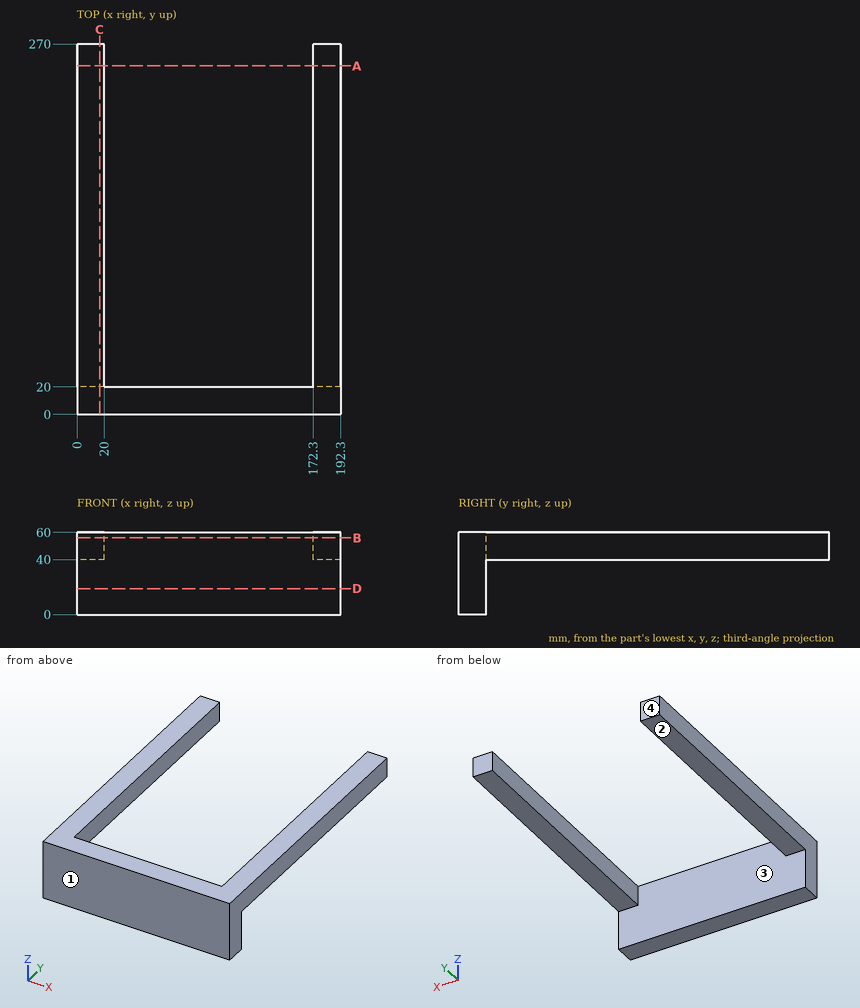
Study the drawing (mm; zero at the part's minimum x, y, z) and answer. A direction names the side the tool comes from. Round coordinates to 2 decimals unless told otherwise and drop trailing zeros. Write each loop counter-clockwise with the first axis right and the second up, starting at its lowest first coordinate (ties: lowest second). Pieces come first, ordered by that corner, then holes. Notation, with made-up numbers: (31.25, 9) - (63.25, 9) arc R19 ccw to (63.25, 18) - close; hole circle Ø11 at (48, 12.5). An arc over 180 degrees is marked (long way). Use a Markdown table: item, result. Add a question column.
1. The part is cut by section A-A (y = 254). Write down the section's boundary in (x, z).
2. Flat-ended cylindrical pins translate along their axes: P1, Ø8, axis at y = 37.5, z = 33.5, coming from the -X side; P2, Ø10, axis at x = 11, y = 160, coming from the -Z side; P3, Ø2, axis at x = 24, z = 51.5, coming from the +Y side. Find the tip coordinate at first contact, or state that the pin passes through.
3. The part is cut by section D-D (z = 19). Write down the section's boundary in (x, y).
4. For a pull along X with two mould halves and no side action, classify the marked faces 3 and 4 as +X half, -X half, draft (parallel to the pull), parting line (faces both ways), or undercut.
5. A tool of negligible diameter and unlimited length cuts with its end or side. For the marked faces 1 and 2, from which of +Z, -Z, +X, -X, +Y, -Y can it reach the whole face along a straight path? Write none if from no direction.
6. Consider line 1 (X direction, y = 44, z = 50); line 2 (Y direction, x = 148.5, z = 38); line 3 (Z direction, x = 176.5, y = 211). Determine where each line is inside the solid, lowest interval first.
7. The part is cut by section C-C (x = 16.5). Write down the section's boundary in (y, z), and give its area (3 significant figures).
8. The part is cut by section B-B (z = 56). Write down the section's boundary in (x, y), and give its area (3 significant figures).
Reported:
| question | item | result |
|---|---|---|
| 1 | outline | (0, 40) - (20, 40) - (20, 60) - (0, 60) - close; (172.3, 40) - (192.3, 40) - (192.3, 60) - (172.3, 60) - close |
| 2 | P1 | through |
| 2 | P2 | z = 40 |
| 2 | P3 | y = 20 |
| 3 | outline | (0, 0) - (192.3, 0) - (192.3, 20) - (0, 20) - close |
| 4 | face 3 | undercut |
| 4 | face 4 | draft |
| 5 | face 1 | +Z, -Z, +X, -X, -Y |
| 5 | face 2 | -Z, +X, -X, +Y |
| 6 | line 1 | 0 to 20, 172.3 to 192.3 |
| 6 | line 2 | 0 to 20 |
| 6 | line 3 | 40 to 60 |
| 7 | outline | (0, 0) - (20, 0) - (20, 40) - (270, 40) - (270, 60) - (0, 60) - close |
| 7 | area | 6,200 mm^2 |
| 8 | outline | (0, 0) - (192.3, 0) - (192.3, 270) - (172.3, 270) - (172.3, 20) - (20, 20) - (20, 270) - (0, 270) - close |
| 8 | area | 13,800 mm^2 |
